The model under review builds one solid part; all positions refer to its coordinate system, in mm. Face numbers are marked on the shaded views. A direction names the side the tool comes from. Round coordinates to 2 decimals unless told otherwise and drop trailing zeros. Write each loop counter-clockwise with the first axis right and the second up, starting at its lowest first coordinate (ties: lowest second). Pieces come first, ordered by that corner, then holes. Notation, with made-up numbers: (21.25, 25.5) -> (68.25, 25.5) arc R23 cw to (68.25, 41.5) -> close; hole circle Ø6 at (19, -32). An arc over 180 degrees is marked (long way). Answer as a JSON object with one key per item and string values. Group by question number.
1) We need section A-A, the plane z = -31.5. Write out the cut boundary in (x, y), then the cut area to 3 significant figures.
2) Mouldability with a two-part tool opening along X and no side actions: class the marked faces 1 and 2 as pulls with the +X half, pulls with the -X half, needs draft (parallel to the pull), parting line crosses it, or undercut.
3) We need section C-C, the plane y = -9.75. Write out the cut boundary in (x, z).
4) We need section B-B, the plane x = 90. Write out the cut boundary in (y, z), then the cut area to 3 significant figures.
5) Insertion check: pin 1 Ø8 at (x, z) = (158, -39) entering from -Y; pin 2 Ø1.5 at (y, z) = (-7.5, -19) entering from +X; pin 3 Ø6 at (x, y) = (145, -12.5) entering from +Z. Each pin has a flat end and moves straight along its axis. Give the tip position at first contact, or say it passes through.
6) Machinability: for the marked faces 3 and 4, which of the approach directions +Z, -Z, +X, -X, +Y, -Y give a long, thin tool a straight path to every point of the face, cutting with its end or side? Answer none if there is none.
7) We need section D-D, the plane x = 30. Write out the cut boundary in (y, z), then the cut area to 3 significant figures.
8) To check wall thickness, follow probe 1 along Z at (x, y) = (90, -2.5); probe 2 along Y at (x, z) = (62.5, -24); probe 3 along Y at (x, z) = (78, -34.5). State the ranges of each line that lie inside material, in increasing order. Write a range as [from, to].
from build123d import *

# Parameters (mm, degrees)
F0_W     = 180
F0_H     = 63
F1_DEPTH = 4
F2_R     = 27
F3_DEPTH = 4
F2_R_2   = 6
F4_DEPTH = 15
F5_SIZE  = 2
F6_R     = 4.9
F7_DEPTH = 25


with BuildPart() as f1:
    # F0 (on Front) → F1 (new body)
    with BuildSketch(Plane.XZ):
        with Locations((90, -31.5)):
            Rectangle(F0_W, F0_H)
    extrude(amount=F1_DEPTH)

    # F2 (on face) → F3 (join)
    with BuildSketch(Plane.XZ.offset(4)):
        with Locations((90, -31.5)):
            Circle(F2_R)
    extrude(amount=F3_DEPTH)

    # F2 (on face) → F4 (join)
    with BuildSketch(Plane.XZ.offset(4)):
        with Locations((30, -7.5)):
            Circle(F2_R_2)
        with Locations((150, -7.5)):
            Circle(F2_R_2)
    extrude(amount=F4_DEPTH)

    # F5
    f5_edges = [f1.edges().sort_by_distance(p)[0] for p in [
        (24, -19, -7.5),
        (144, -19, -7.5),
    ]]
    chamfer(f5_edges, length=F5_SIZE)

    # F6 (on face) → F7 (cut)
    with BuildSketch(Plane.XZ.offset(8)):
        with Locations((90, -31.5)):
            Circle(F6_R)
    extrude(amount=-F7_DEPTH, mode=Mode.SUBTRACT)


solid = f1.part
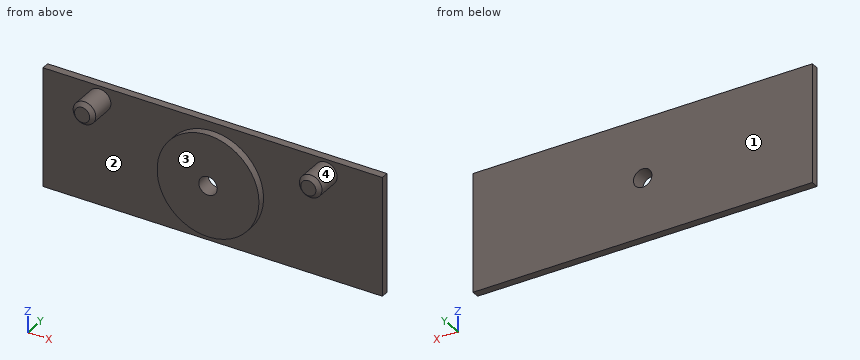
Here are the results:
{
 "1": {"outline": "(0, -4) -> (63, -4) -> (63, -8) -> (85.1, -8) -> (85.1, 0) -> (0, 0) -> close; (94.9, -8) -> (117, -8) -> (117, -4) -> (180, -4) -> (180, 0) -> (94.9, 0) -> close", "area": "858 mm^2"},
 "2": {"face 1": "needs draft", "face 2": "undercut"},
 "3": {"outline": "circle Ø12 at (30, -7.5); circle Ø12 at (150, -7.5)"},
 "4": {"outline": "(-8, -58.5) -> (-4, -58.5) -> (-4, -63) -> (0, -63) -> (0, -36.4) -> (-8, -36.4) -> close; (-8, -26.6) -> (0, -26.6) -> (0, 0) -> (-4, 0) -> (-4, -4.5) -> (-8, -4.5) -> close", "area": "390 mm^2"},
 "5": {"pin 1": "stops at y = -4", "pin 2": "stops at x = 114.31", "pin 3": "stops at z = -1.84"},
 "6": {"face 3": "+Z, -Z, -Y", "face 4": "-Y"},
 "7": {"outline": "(-19, -11.5) -> (-17, -13.5) -> (-4, -13.5) -> (-4, -63) -> (0, -63) -> (0, 0) -> (-4, 0) -> (-4, -1.5) -> (-17, -1.5) -> (-19, -3.5) -> close", "area": "428 mm^2"},
 "8": {"probe 1": "z = [-63, -36.4], [-26.6, 0]", "probe 2": "y = [-4, 0]", "probe 3": "y = [-8, 0]"}
}
